from build123d import *

# Parameters (mm, degrees)
F0_R     = 2
F0_R_2   = 17.5
F1_DEPTH = 2
F2_R     = 3
F3_R     = 5


with BuildPart() as f1:
    # F0 (on Top) → F1 (new body)
    with BuildSketch(Plane.XY):
        with BuildLine():
            Line((-10, 22), (-10, 17.89553))
            ThreePointArc((-10, 17.89553), (-20.353721, -2.444595), (-5.478019, -19.754526))
            Line((-5.478019, -19.754526), (-4.980973, -25.435779))
            ThreePointArc((-4.980973, -25.435779), (0, -30), (4.980973, -25.435779))
            Line((4.980973, -25.435779), (5.478019, -19.754526))
            ThreePointArc((5.478019, -19.754526), (20.353721, -2.444595), (10, 17.89553))
            Line((10, 17.89553), (10, 22))
            Line((10, 22), (-10, 22))
        make_face()
        with Locations((0, -25)):
            Circle(F0_R, mode=Mode.SUBTRACT)
        Circle(F0_R_2, mode=Mode.SUBTRACT)
    extrude(amount=F1_DEPTH)

    # F2
    f2_edges = [f1.edges().sort_by_distance(p)[0] for p in [
        (-10, 22, 1),
        (10, 22, 1),
        (-5.478019, -19.754526, 1),
        (5.478019, -19.754526, 1),
    ]]
    fillet(f2_edges, radius=F2_R)

    # F3
    f3_edges = [f1.edges().sort_by_distance(p)[0] for p in [
        (-10, 17.89553, 1),
        (10, 17.89553, 1),
    ]]
    fillet(f3_edges, radius=F3_R)


solid = f1.part
Could you check a few things on this model? Use its own coordinates, in mm. Round coordinates to 2 decimals unless told otherwise and drop trailing zeros. Write each loop counter-clockwise with the first axis right and the second up, starting at its lowest first coordinate (ties: lowest second). Pieces come first, ordered by that corner, then holes. Notation, with made-up numbers: (80.5, 61.25) - (113.5, 61.25) arc R14 cw to (113.5, 80.25) - close; hole circle Ø5 at (-7, -16.5). An arc over 180 degrees is marked (long way). Put each result on its own line as item: value. Start each with the question number.
(1) Thinking about a two-plate mould opening in Y: for faces 1 (the cylindrical face through (0.923, -26.774, 0.986)), 2 (the flat face through (0, 22, 1)), 3 (the cylindrical face through (-5.918, -20.157, 1.014)), 4 (the flat face through (4.5, -17.4, 2)), which applies, released by +Y, released by -Y, zero draft, split by the parting line, or undercut?
(2) I need wall thicknesses on probe 1 along Y at (x, z) = (0, 1.15); probe 2 along X at (y, z) = (0.5, 0.6); probe 3 along Y at (x, z) = (-4, 1.2). Which ranges of each line are inside material? Lowest first, please.
(3) I want a section at D-D, the plane z = 0.5. Give the number of separate pieces and of enclosed holes in the cut face, plus the area to 3 significant figures.
(4) I want a section at B-B, the plane y = 4.5. Please give me the cut outline in (x, z).
(5) I want a section at C-C, the plane y = 10. Please give me the cut outline in (x, z), plus the area to 3 significant figures.
(6) I want a section at A-A, the plane x = 0. Please give me the cut outline in (y, z).
Here are the results:
1. face 1: undercut
1. face 2: released by +Y
1. face 3: released by -Y
1. face 4: zero draft
2. probe 1: y = -30 to -27, -23 to -17.5, 17.5 to 22
2. probe 2: x = -20.49 to -17.49, 17.49 to 20.49
2. probe 3: y = -28 to -17.04, 17.04 to 22
3. separate pieces: 1
3. enclosed holes: 2
3. area: 480 mm^2
4. outline: (-20, 0) - (-16.91, 0) - (-16.91, 2) - (-20, 2) - close; (16.91, 0) - (20, 0) - (20, 2) - (16.91, 2) - close
5. outline: (-17.9, 0) - (-14.36, 0) - (-14.36, 2) - (-17.9, 2) - close; (14.36, 0) - (17.9, 0) - (17.9, 2) - (14.36, 2) - close
5. area: 14.1 mm^2
6. outline: (-30, 0) - (-27, 0) - (-27, 2) - (-30, 2) - close; (-23, 0) - (-17.5, 0) - (-17.5, 2) - (-23, 2) - close; (17.5, 0) - (22, 0) - (22, 2) - (17.5, 2) - close
